from build123d import *

# Parameters (mm, degrees)
BOSS_EXTRUDE1_DEPTH      = 15
BOSS_EXTRUDE1_DEPTH_BACK = 15
CUT_EXTRUDE1_REACH       = 22.368
SKETCH2_R                = 2.15
CUT_EXTRUDE2_REACH       = 26.368
CUT_EXTRUDE2_START       = -4
SKETCH3_R                = 3.25


with BuildPart() as part:
    # Sketch1 → Boss-Extrude1 (new body, two sides)
    with BuildSketch(Plane(origin=(0, 0, 0), x_dir=(1, 0, 0), z_dir=(0, 1, 0))) as boss_extrude1_sk:
        with BuildLine():
            Line((-9.9, 6.5), (-9.9, 0))
            ThreePointArc((-9.9, 0), (-7.277705682, -6.711557196), (-0.8, -9.867623827))
            Line((-0.8, -9.867623827), (-0.8, -7.457211275))
            ThreePointArc((-0.8, -7.457211275), (0, 7.5), (0.8, -7.457211275))
            Line((0.8, -7.457211275), (0.8, -9.867623827))
            ThreePointArc((0.8, -9.867623827), (7.277705682, -6.711557196), (9.9, 0))
            Line((9.9, 0), (9.9, 6.5))
            Line((9.9, 6.5), (17, 6.5))
            Line((17, 6.5), (17, 10.5))
            Line((17, 10.5), (-17, 10.5))
            Line((-17, 10.5), (-17, 6.5))
            Line((-17, 6.5), (-9.9, 6.5))
        make_face()
    extrude(amount=BOSS_EXTRUDE1_DEPTH)
    extrude(boss_extrude1_sk.sketch, amount=-BOSS_EXTRUDE1_DEPTH_BACK)

    # Sketch2 → Cut-Extrude1 (cut, up to next)
    with BuildSketch(Plane(origin=(0, 0, -10.5), x_dir=(-1, 0, 0), z_dir=(0, 0, -1)), mode=Mode.PRIVATE) as cut_extrude1_sk1:
        with Locations((12, -9)):
            Circle(SKETCH2_R)
    cut_extrude1_tool1 = extrude(cut_extrude1_sk1.sketch, amount=-CUT_EXTRUDE1_REACH, mode=Mode.PRIVATE) & part.part
    add(cut_extrude1_tool1.solids().sort_by_distance((-12, -9, -10.5))[0], mode=Mode.SUBTRACT)
    # Sketch2 → Cut-Extrude1 (cut, up to next)
    with BuildSketch(Plane(origin=(0, 0, -10.5), x_dir=(-1, 0, 0), z_dir=(0, 0, -1)), mode=Mode.PRIVATE) as cut_extrude1_sk2:
        with Locations((-12, -9)):
            Circle(SKETCH2_R)
    cut_extrude1_tool2 = extrude(cut_extrude1_sk2.sketch, amount=-CUT_EXTRUDE1_REACH, mode=Mode.PRIVATE) & part.part
    add(cut_extrude1_tool2.solids().sort_by_distance((12, -9, -10.5))[0], mode=Mode.SUBTRACT)
    # Sketch2 → Cut-Extrude1 (cut, up to next)
    with BuildSketch(Plane(origin=(0, 0, -10.5), x_dir=(-1, 0, 0), z_dir=(0, 0, -1)), mode=Mode.PRIVATE) as cut_extrude1_sk3:
        with Locations((-12, 9)):
            Circle(SKETCH2_R)
    cut_extrude1_tool3 = extrude(cut_extrude1_sk3.sketch, amount=-CUT_EXTRUDE1_REACH, mode=Mode.PRIVATE) & part.part
    add(cut_extrude1_tool3.solids().sort_by_distance((12, 9, -10.5))[0], mode=Mode.SUBTRACT)
    # Sketch2 → Cut-Extrude1 (cut, up to next)
    with BuildSketch(Plane(origin=(0, 0, -10.5), x_dir=(-1, 0, 0), z_dir=(0, 0, -1)), mode=Mode.PRIVATE) as cut_extrude1_sk4:
        with Locations((12, 9)):
            Circle(SKETCH2_R)
    cut_extrude1_tool4 = extrude(cut_extrude1_sk4.sketch, amount=-CUT_EXTRUDE1_REACH, mode=Mode.PRIVATE) & part.part
    add(cut_extrude1_tool4.solids().sort_by_distance((-12, 9, -10.5))[0], mode=Mode.SUBTRACT)

    # Sketch3 → Cut-Extrude2 (cut, up to next)
    with BuildSketch(Plane(origin=(0, 0, -10.5), x_dir=(-1, 0, 0), z_dir=(0, 0, -1)).offset(CUT_EXTRUDE2_START), mode=Mode.PRIVATE) as cut_extrude2_sk1:
        with Locations((-12, 9)):
            Circle(SKETCH3_R)
    cut_extrude2_tool1 = extrude(cut_extrude2_sk1.sketch, amount=-CUT_EXTRUDE2_REACH, mode=Mode.PRIVATE) & part.part
    add(cut_extrude2_tool1.solids().sort_by_distance((12, 9, -6.5))[0], mode=Mode.SUBTRACT)
    # Sketch3 → Cut-Extrude2 (cut, up to next)
    with BuildSketch(Plane(origin=(0, 0, -10.5), x_dir=(-1, 0, 0), z_dir=(0, 0, -1)).offset(CUT_EXTRUDE2_START), mode=Mode.PRIVATE) as cut_extrude2_sk2:
        with Locations((-12, -9)):
            Circle(SKETCH3_R)
    cut_extrude2_tool2 = extrude(cut_extrude2_sk2.sketch, amount=-CUT_EXTRUDE2_REACH, mode=Mode.PRIVATE) & part.part
    add(cut_extrude2_tool2.solids().sort_by_distance((12, -9, -6.5))[0], mode=Mode.SUBTRACT)
    # Sketch3 → Cut-Extrude2 (cut, up to next)
    with BuildSketch(Plane(origin=(0, 0, -10.5), x_dir=(-1, 0, 0), z_dir=(0, 0, -1)).offset(CUT_EXTRUDE2_START), mode=Mode.PRIVATE) as cut_extrude2_sk3:
        with Locations((12, 9)):
            Circle(SKETCH3_R)
    cut_extrude2_tool3 = extrude(cut_extrude2_sk3.sketch, amount=-CUT_EXTRUDE2_REACH, mode=Mode.PRIVATE) & part.part
    add(cut_extrude2_tool3.solids().sort_by_distance((-12, 9, -6.5))[0], mode=Mode.SUBTRACT)
    # Sketch3 → Cut-Extrude2 (cut, up to next)
    with BuildSketch(Plane(origin=(0, 0, -10.5), x_dir=(-1, 0, 0), z_dir=(0, 0, -1)).offset(CUT_EXTRUDE2_START), mode=Mode.PRIVATE) as cut_extrude2_sk4:
        with Locations((12, -9)):
            Circle(SKETCH3_R)
    cut_extrude2_tool4 = extrude(cut_extrude2_sk4.sketch, amount=-CUT_EXTRUDE2_REACH, mode=Mode.PRIVATE) & part.part
    add(cut_extrude2_tool4.solids().sort_by_distance((-12, -9, -6.5))[0], mode=Mode.SUBTRACT)


solid = part.part
Model file for the job. Use its own axes, mm. A direction names the side the tool comes from. Round coordinates to 2 decimals unless told otherwise and drop trailing zeros. Loops run counter-clockwise (first coordinate to the right, second up) from the corner with the lowest first, then second, coordinate; pieces in that order, holes last.
1. Band-saw the part on B-B, the plane x = 12. List the corners of the cut face in (y, z), and give its area (3 significant figures).
Check values:
outline: (-15, -10.5) - (-11.15, -10.5) - (-11.15, -6.5) - (-15, -6.5) - close; (-6.85, -10.5) - (6.85, -10.5) - (6.85, -6.5) - (-6.85, -6.5) - close; (11.15, -10.5) - (15, -10.5) - (15, -6.5) - (11.15, -6.5) - close
area: 85.6 mm2
2. Tool access for faces 4 (the flat face through (0.8, 0, 9)), 5 (the cylindrical face through (-8.75, -8.96, -1.01)), 6 (the cylindrical face through (8.75, 8.96, -1.01)), 7 (the flat face through (-9.9, -13, -3)), 8 (the flat face through (9.9, 13, -3)): list every direction of +Z, -Z, +X, -X, +Y, -Y with a clear straight run to the whole face (end or side of a thin tool).
Check values:
face 4: +Z, +Y, -Y
face 5: +Z, -X
face 6: +Z, +X
face 7: +Z, -X, +Y, -Y
face 8: +Z, +X, +Y, -Y
3. Mould opens along X. For faces 1 (the flat face through (-14, 0, -6.5)), 2 (the flat face through (-0.8, 0, 9)), 3 (the flat face through (-17, 0, -9)) say: +X half, -X half, draft (parallel to the pull), parting line (faces both ways), or undercut.
Check values:
face 1: draft
face 2: undercut
face 3: -X half
4. Band-saw the part on D-D, the plane z = -4. List the corners of the cut face in (x, y), and give its area (3 significant figures).
Check values:
outline: (-9.9, -15) - (-6.34, -15) - (-6.34, 15) - (-9.9, 15) - (-9.9, 11.48) arc R3.25 cw to (-9.9, 6.52) - (-9.9, -6.52) arc R3.25 cw to (-9.9, -11.48) - close; (6.34, -15) - (9.9, -15) - (9.9, -11.48) arc R3.25 cw to (9.9, -6.52) - (9.9, 6.52) arc R3.25 cw to (9.9, 11.48) - (9.9, 15) - (6.34, 15) - close
area: 197 mm2
5. Wall check: probe 1 along Y at (x, z) = (-12, -8.95); probe 2 along Y at (x, z) = (13.5, -8.25); probe 3 along Z at (x, y) = (10, -14). Give the ranges that are in metal, low to high.
Check values:
probe 1: y = -15 to -11.15, -6.85 to 6.85, 11.15 to 15
probe 2: y = -15 to -10.54, -7.46 to 7.46, 10.54 to 15
probe 3: z = -10.5 to -6.5
6. Band-saw the part on C-C, the plane y = 12. List the corners of the cut face in (x, z).
Check values:
outline: (-17, -10.5) - (17, -10.5) - (17, -6.5) - (9.9, -6.5) - (9.9, 0) arc R9.9 ccw to (0.8, 9.87) - (0.8, 7.46) arc R7.5 cw (long way) to (-0.8, 7.46) - (-0.8, 9.87) arc R9.9 ccw to (-9.9, 0) - (-9.9, -6.5) - (-17, -6.5) - close
7. Band-saw the part on A-A, the plane y = -9. List the corners of the cut face in (x, z), and give its area (3 significant figures).
Check values:
outline: (-17, -10.5) - (-14.15, -10.5) - (-14.15, -6.5) - (-17, -6.5) - close; (-9.85, -10.5) - (9.85, -10.5) - (9.85, -6.5) - (8.75, -6.5) - (8.75, 4.63) arc R9.9 ccw to (0.8, 9.87) - (0.8, 7.46) arc R7.5 cw (long way) to (-0.8, 7.46) - (-0.8, 9.87) arc R9.9 ccw to (-8.75, 4.63) - (-8.75, -6.5) - (-9.85, -6.5) - close; (14.15, -10.5) - (17, -10.5) - (17, -6.5) - (14.15, -6.5) - close
area: 182 mm2
8. Drop flat-ended pins along their axis: P1, Ø5.5, axis at x = 12, y = 9, coming from the +Z side; P2, Ø3, axis at y = 3, z = 4.5, coming from the +X side; P3, Ø0.7, axis at y = -6.5, z = 8.5, coming from the +X side. Give the stop position or say it passes through.
Check values:
P1: stops at z = -6.5
P2: stops at x = 9.43
P3: stops at x = 5.62
